Check sheet for the modelled part. Datum: model origin and axes. Units: mm. A direction names the side the tool comes from. Round coordinates to 2 decimals unless told otherwise and drop trailing zeros. Loops run counter-clockwise (first coordinate to the right, second up) from the corner with the lowest first, then second, coordinate; pieces in that order, holes last. Notation, with made-up numbers: (-36.75, 88.25) -> (-31.75, 88.25) arc R32 cw to (-31.75, 117.25) -> close; hole circle Ø5 at (33, -26). An arc over 180 degrees is marked (long way). Return JSON: item names as keys, results as strings.
from build123d import *

# Parameters (mm, degrees)
F0_R         = 25
F1_DEPTH     = 7
F2_R         = 5
F3_DEPTH     = 6
F5_DEPTH     = 8
F7_R         = 25
F7_R_2       = 24.4
F8_DEPTH     = 5
F10_DEPTH    = 25
F11_R        = 5
F12_T1_DEPTH = 7
F13_R        = 2


# Not quite as in the source:
# - a fillet or chamfer that OpenCascade refuses, or shapes differently, is made with other operations: its cross-section is extruded or revolved along the edge and cut away or added


with BuildPart() as f1:
    # F0 (on Top) → F1 (new body)
    with BuildSketch(Plane.XY):
        Circle(F0_R)
    extrude(amount=F1_DEPTH)

    # F2 (on face) → F3 (join)
    with BuildSketch(Plane.XY.offset(7)):
        Circle(F2_R)
    extrude(amount=F3_DEPTH)

    # F4 (on face) → F5 (cut)
    with BuildSketch(Plane.XY.offset(13)):
        with BuildLine():
            Line((2.1498313887, 1.825), (-2.1498313887, 1.825))
            ThreePointArc((-2.1498313887, 1.825), (-2.82, 0), (-2.1498313887, -1.825))
            Line((-2.1498313887, -1.825), (2.1498313887, -1.825))
            ThreePointArc((2.1498313887, -1.825), (2.82, 0), (2.1498313887, 1.825))
        make_face()
    extrude(amount=-F5_DEPTH, mode=Mode.SUBTRACT)

    # F7 (on offset) → F8 (cut)
    with BuildSketch(Plane.XY.offset(1)):
        Circle(F7_R)
        Circle(F7_R_2, mode=Mode.SUBTRACT)
    extrude(amount=F8_DEPTH, mode=Mode.SUBTRACT)

    # F9 (on face) → F10 (cut)
    with BuildSketch(Plane.XY.offset(7)):
        with BuildLine():
            Line((7.1352549156, 7.0062926922), (15.9346604169, 12.0866318271))
            ThreePointArc((15.9346604169, 12.0866318271), (0, 20.0000017881), (-15.9346604169, 12.0866318271))
            Line((-15.9346604169, 12.0866318271), (-7.1352549156, 7.0062926922))
            ThreePointArc((-7.1352549156, 7.0062926922), (0, 10), (7.1352549156, 7.0062926922))
        make_face()
        with BuildLine():
            ThreePointArc((2.5, -19.8431366353), (15.0000012666, -13.2287578225), (20.0000017881, 0))
            ThreePointArc((20.0000017881, 0), (19.6047610649, 3.9564397015), (18.4346604169, 7.7565048082))
            Line((18.4346604169, 7.7565048082), (9.6352549156, 2.6761656733))
            ThreePointArc((9.6352549156, 2.6761656733), (9.9083941473, 1.3504537837), (10, 0))
            ThreePointArc((10, 0), (7.9056941504, -6.123724357), (2.5, -9.6824583655))
            Line((2.5, -9.6824583655), (2.5, -19.8431366353))
        make_face()
        with BuildLine():
            ThreePointArc((-18.4346604169, 7.7565048082), (-17.3205096243, -10.0000008941), (-2.5, -19.8431366353))
            Line((-2.5, -19.8431366353), (-2.5, -9.6824583655))
            ThreePointArc((-2.5, -9.6824583655), (-8.6602540378, -5), (-9.6352549156, 2.6761656733))
            Line((-9.6352549156, 2.6761656733), (-18.4346604169, 7.7565048082))
        make_face()
    extrude(amount=-F10_DEPTH, mode=Mode.SUBTRACT)

    # F11
    f11_edges = [f1.edges().sort_by_distance(p)[0] for p in [
        (-18.43466, 7.756505, 3.5),
        (-15.93466, 12.086632, 3.5),
        (15.93466, 12.086632, 3.5),
        (18.43466, 7.756505, 3.5),
        (2.5, -19.843137, 3.5),
        (-2.5, -19.843137, 3.5),
    ]]
    fillet(f11_edges, radius=F11_R)

    # F12: fillet of radius 5 on 6 edges, made by hand

    # F12_s2 → F12_t1 (join)
    with BuildSketch(Plane.XY):
        with BuildLine():
            ThreePointArc((-12.5, 4.3301270189), (-10.6698729811, 2.5), (-10, 0))
            ThreePointArc((-10, 0), (-9.9083941473, 1.3504537837), (-9.6352549156, 2.6761656733))
            Line((-9.6352549156, 2.6761656733), (-12.5, 4.3301270189))
        make_face()
        with BuildLine():
            ThreePointArc((-2.5, -12.9903810568), (-3.1698729811, -10.4903810568), (-5, -8.6602540378))
            ThreePointArc((-5, -8.6602540378), (-3.7846697903, -9.2561479341), (-2.5, -9.6824583655))
            Line((-2.5, -9.6824583655), (-2.5, -12.9903810568))
        make_face()
        with BuildLine():
            ThreePointArc((2.5, -12.9903810568), (3.1698729811, -10.4903810568), (5, -8.6602540378))
            ThreePointArc((5, -8.6602540378), (3.7846697903, -9.2561479341), (2.5, -9.6824583655))
            Line((2.5, -9.6824583655), (2.5, -12.9903810568))
        make_face()
        with BuildLine():
            ThreePointArc((12.5, 4.3301270189), (10.6698729811, 2.5), (10, 0))
            ThreePointArc((10, 0), (9.9083941473, 1.3504537837), (9.6352549156, 2.6761656733))
            Line((9.6352549156, 2.6761656733), (12.5, 4.3301270189))
        make_face()
        with BuildLine():
            ThreePointArc((10, 8.6602540378), (7.5, 7.9903810568), (5, 8.6602540378))
            ThreePointArc((5, 8.6602540378), (6.123724357, 7.9056941504), (7.1352549156, 7.0062926922))
            Line((7.1352549156, 7.0062926922), (10, 8.6602540378))
        make_face()
        with BuildLine():
            ThreePointArc((-10, 8.6602540378), (-7.5, 7.9903810568), (-5, 8.6602540378))
            ThreePointArc((-5, 8.6602540378), (-6.123724357, 7.9056941504), (-7.1352549156, 7.0062926922))
            Line((-7.1352549156, 7.0062926922), (-10, 8.6602540378))
        make_face()
    extrude(amount=F12_T1_DEPTH)

    # F13
    f13_edges = [f1.edges().sort_by_distance(p)[0] for p in [
        (-5, 0, 7),
        (-5, 0, 13),
    ]]
    fillet(f13_edges, radius=F13_R)


solid = f1.part
Q1. Draft check along Y on faces 1 (the cylindrical face through (-1.08, -4.88, 9.99)), 2 (the flat face through (0, -2, 13)), 3 (the cylindrical face through (-2.82, 0.03, 9.06)), 4 (the cylindrical face through (3.152, -10.522, 3.451)). Enter one of: released by +Y, released by -Y, zero draft, split by the parting line, or undercut.
Results list:
{"face 1": "split by the parting line", "face 2": "zero draft", "face 3": "undercut", "face 4": "undercut"}
Q2. Section check A-A (x = 0). Record the boundary of the cut face in (y, z) (3 decimals), then the cut area to 3 significant figures.
Results list:
{"outline": "(-25, 0) -> (10, 0) -> (10, 7) -> (7, 7) arc R2 cw to (5, 9) -> (5, 11) arc R2 ccw to (3, 13) -> (1.825, 13) -> (1.825, 5) -> (-1.825, 5) -> (-1.825, 13) -> (-3, 13) arc R2 ccw to (-5, 11) -> (-5, 9) arc R2 cw to (-7, 7) -> (-25, 7) -> (-25, 6) -> (-24.4, 6) -> (-24.4, 1) -> (-25, 1) -> close; (20, 0) -> (25, 0) -> (25, 1) -> (24.4, 1) -> (24.4, 6) -> (25, 6) -> (25, 7) -> (20, 7) -> close", "area": "305 mm^2"}
Q3. Material ranges on line 1 (Y direction, x = -0.5, z = 6.25) (1 decimal); line 2 (Y direction, x = -0.5, z = 3); line 3 (Y direction, x = -4, z = 5.25), recorded low to high.
Results list:
{"line 1": "-25 to -1.8, 1.8 to 10, 20 to 25", "line 2": "-24.39 to 9.99, 19.99 to 24.39", "line 3": "-24.07 to -16.56, -9.42 to 9.17, 19.6 to 24.07"}
Q4. Tool access check on faces 5 (the cylindrical face through (7.54, 7.99, 3.45)), 6 (the flat face through (24, -5.4, 6)), 7 (the cylindrical face through (2.82, -0.03, 9.06)). Record the directions out of +Z, -Z, +X, -X, +Y, -Y that give a thin tool (end or side, any length) a straight path to the whole face; none if there is none.
Results list:
{"face 5": "+Z, -Z", "face 6": "none", "face 7": "+Z"}
Q5. Section check C-C (y = 11). Record the boundary of the cut face in (x, z), then the cut area to 3 significant figures.
Results list:
{"outline": "(-22.45, 0) -> (-12.09, 0) -> (-12.09, 7) -> (-22.45, 7) -> (-22.45, 6) -> (-21.78, 6) -> (-21.78, 1) -> (-22.45, 1) -> close; (12.09, 0) -> (22.45, 0) -> (22.45, 1) -> (21.78, 1) -> (21.78, 6) -> (22.45, 6) -> (22.45, 7) -> (12.09, 7) -> close", "area": "138 mm^2"}
Q6. Section check D-D (x = -8). Record the boundary of the cut face in (y, z), then the cut area to 3 significant figures.
Results list:
{"outline": "(-23.69, 0) -> (-17.97, 0) -> (-17.97, 7) -> (-23.69, 7) -> (-23.69, 6) -> (-23.05, 6) -> (-23.05, 1) -> (-23.69, 1) -> close; (-6, 0) -> (8.02, 0) -> (8.02, 7) -> (-6, 7) -> close; (18.33, 0) -> (23.69, 0) -> (23.69, 1) -> (23.05, 1) -> (23.05, 6) -> (23.69, 6) -> (23.69, 7) -> (18.33, 7) -> close", "area": "169 mm^2"}
Q7. Go/stop test with flat-tipped pins: pin 1 (4 mm diameter, centred on x = 18, y = 8, fed in from -Z); pin 2 (4.5 mm diameter, centred on x = -0.5, z = 11, fed in from +Y); pin 3 (3 mm diameter, centred on y = 20, z = 5, fed in from +X); pin 4 (1.8 mm diameter, centred on x = -1, y = -0.5, fed in from +Z). Record where each tip stops, or that it passes through.
Results list:
{"pin 1": "z = 0", "pin 2": "y = 5.01", "pin 3": "x = 16.39", "pin 4": "z = 5"}
